Check sheet for the modelled part. Datum: model origin and axes. Units: mm. A direction names the side the tool comes from. Give positions to 0.01 mm unless a question says otherwise; leave off trailing zeros. Write each loop counter-clockwise with the first axis right and the second up, starting at its lowest first coordinate (ties: lowest second). Pieces come first, ordered by that corner, then holes. Notation, with made-up numbers: M 80.25,0 L 112.25,0 A16 ccw 112.25,11 Z; hole C 15,9.25 d8. An arc over 180 degrees is marked long. One line per item, written item: value. Start each with the question number.
from build123d import *

# Parameters (mm, degrees)
CROQUIS1_W                         = 80
CROQUIS1_H                         = 190
BRIDA_BASE1_DEPTH                  = 3
BRIDA_DE_ARISTA1_STRIP_W           = 15
BRIDA_DE_ARISTA1_STRIP_H           = 3
BRIDA_DE_ARISTA1_STRIP_CUT_DEPTH   = 190
BRIDA_DE_ARISTA1_STRIP_2_W         = 15
BRIDA_DE_ARISTA1_STRIP_2_H         = 3
BRIDA_DE_ARISTA1_STRIP_CUT_2_DEPTH = 190
BRIDA_DE_ARISTA1_DEPTH             = 190
BRIDA_DE_ARISTA1_BEND_DEPTH        = 190
TALADRO_DE_MARGEN_PARA_M61_D       = 6.6
TALADRO_DE_MARGEN_PARA_M61_DEPTH   = 500
TALADRO_DE_MARGEN_PARA_M61_TIP     = 1.982840043
REDONDEO2_R                        = 10


# Sheet-metal steps are written as plain solids
with BuildPart() as part:
    # Croquis1 → Brida base1 (new body)
    with BuildSketch(Plane.XY):
        Rectangle(CROQUIS1_W, CROQUIS1_H)
    extrude(amount=-BRIDA_BASE1_DEPTH)

    # Brida de arista1 strip (across the edge) → Brida de arista1 strip cut (cut)
    with BuildSketch(Plane(origin=(-40, 95, 0), x_dir=(1, 0, 0), z_dir=(0, -1, 0))):
        with Locations((-6, -1.5)):
            Rectangle(BRIDA_DE_ARISTA1_STRIP_W, BRIDA_DE_ARISTA1_STRIP_H)
    extrude(amount=BRIDA_DE_ARISTA1_STRIP_CUT_DEPTH, mode=Mode.SUBTRACT)

    # Brida de arista1 strip 2 (across the edge) → Brida de arista1 strip cut 2 (cut)
    with BuildSketch(Plane(origin=(40, -95, 0), x_dir=(-1, 0, 0), z_dir=(0, 1, 0))):
        with Locations((-6, -1.5)):
            Rectangle(BRIDA_DE_ARISTA1_STRIP_2_W, BRIDA_DE_ARISTA1_STRIP_2_H)
    extrude(amount=BRIDA_DE_ARISTA1_STRIP_CUT_2_DEPTH, mode=Mode.SUBTRACT)

    # Brida de arista1 section (across the edge) → Brida de arista1 (add)
    with BuildSketch(Plane(origin=(-40, 95, 0), x_dir=(1, 0, 0), z_dir=(0, -1, 0))):
        with BuildLine():
            Line((-3, 1.5), (-3, 35))
            Line((-3, 35), (0, 35))
            Line((0, 35), (0, 1.5))
            ThreePointArc((0, 1.5), (0.439339828, 0.439339828), (1.5, 0))
            Line((1.5, 0), (1.5, -3))
            ThreePointArc((1.5, -3), (-1.681980515, -1.681980515), (-3, 1.5))
        make_face()
    extrude(amount=BRIDA_DE_ARISTA1_DEPTH)

    # Brida de arista1 section 2 (across the edge) → Brida de arista1 bend (add)
    with BuildSketch(Plane(origin=(40, -95, 0), x_dir=(-1, 0, 0), z_dir=(0, 1, 0))):
        with BuildLine():
            Line((-3, 1.5), (-3, 35))
            Line((-3, 35), (0, 35))
            Line((0, 35), (0, 1.5))
            ThreePointArc((0, 1.5), (0.439339828, 0.439339828), (1.5, 0))
            Line((1.5, 0), (1.5, -3))
            ThreePointArc((1.5, -3), (-1.681980515, -1.681980515), (-3, 1.5))
        make_face()
    extrude(amount=BRIDA_DE_ARISTA1_BEND_DEPTH)

    # Taladro de margen para M61
    with Locations(Plane.XY):
        with Locations((0, 83), (0, -83)):
            Hole(TALADRO_DE_MARGEN_PARA_M61_D / 2, depth=TALADRO_DE_MARGEN_PARA_M61_DEPTH)
            with Locations((0, 0, -(TALADRO_DE_MARGEN_PARA_M61_DEPTH + TALADRO_DE_MARGEN_PARA_M61_TIP / 2))):  # 118° drill point
                Cone(0, TALADRO_DE_MARGEN_PARA_M61_D / 2, TALADRO_DE_MARGEN_PARA_M61_TIP, mode=Mode.SUBTRACT)

    # Redondeo2
    redondeo2_edges = [part.edges().sort_by_distance(p)[0] for p in [
        (-41.5, 95, 35),
        (-41.5, -95, 35),
        (41.5, -95, 35),
        (41.5, 95, 35),
    ]]
    fillet(redondeo2_edges, radius=REDONDEO2_R)


solid = part.part
1) Draft check along Y on faces 3 (the flat face through (-43, 1, 18)), 4 (the cylindrical face through (-1.774, 85.783, -1.521)), 5 (the cylindrical face through (-41.48, -92.15, 31.99)). Enter one of: released by +Y, released by -Y, zero draft, split by the parting line, or undercut.
2) Material ranges on L1, parallel to Y at x = 0, z = -2.25; L2, parallel to X at y = -4, z = 14.5; L3, parallel to Z at x = -23.5, y = 52, recorded low to high. Write a range as from..to.
3) Cross-section at C-C (y = 83). Record the boundary of the cut face in (x, z), plus the area to 3 significant figures.
4) Cross-section at D-D (y = -56.5). Record the boundary of the cut face in (x, z), plus the area to 3 significant figures.
5) Tool access check on faces 1 (the flat face through (43, -1, 18)), 2 (the flat face through (-1, 1, 0)). Record the directions out of +Z, -Z, +X, -X, +Y, -Y that give a thin tool (end or side, any length) a straight path to the whole face; none if there is none.
6) Cross-section at A-A (x = 0). Record the boundary of the cut face in (y, z).
7) Cross-section at B-B (z = 13.5). Record the boundary of the cut face in (x, y), plus the area to 3 significant figures.
8) Gauge pin test, flat ends, axial feed: pin 1 (1 mm diameter, centred on x = 18, y = 4.5, fed in from +Z); pin 2 (7.5 mm diameter, centred on x = 0, y = -83, fed in from -Z). Record the tip position at first contact, or that the pin passes through.
Data:
1. face 3: zero draft
1. face 4: undercut
1. face 5: released by -Y
2. L1: y = -95..-86.3, -79.7..79.7, 86.3..95
2. L2: x = -43..-40, 40..43
2. L3: z = -3..0
3. outline: M -43,1.5 A4.5 ccw -38.5,-3 L -3.3,-3 L -3.3,0 L -38.5,0 A1.5 cw -40,1.5 L -40,35 L -43,35 Z; M 3.3,-3 L 38.5,-3 A4.5 ccw 43,1.5 L 43,35 L 40,35 L 40,1.5 A1.5 cw 38.5,0 L 3.3,0 Z
3. area: 440 mm2
4. outline: M -43,1.5 A4.5 ccw -38.5,-3 L 38.5,-3 A4.5 ccw 43,1.5 L 43,35 L 40,35 L 40,1.5 A1.5 cw 38.5,0 L -38.5,0 A1.5 cw -40,1.5 L -40,35 L -43,35 Z
4. area: 460 mm2
5. face 1: +Z, -Z, +X, +Y, -Y
5. face 2: +Z, +Y, -Y
6. outline: M -95,-3 L -86.3,-3 L -86.3,0 L -95,0 Z; M -79.7,-3 L 79.7,-3 L 79.7,0 L -79.7,0 Z; M 86.3,-3 L 95,-3 L 95,0 L 86.3,0 Z
7. outline: M -43,-95 L -40,-95 L -40,95 L -43,95 Z; M 40,-95 L 43,-95 L 43,95 L 40,95 Z
7. area: 1,140 mm2
8. pin 1: stops at z = 0
8. pin 2: stops at z = -3
